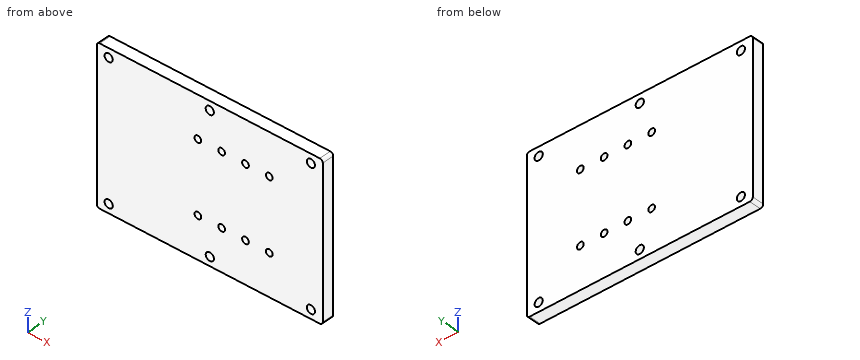
```python
from build123d import *

# Parameters (mm, degrees)
SKETCH1_W               = 482.6
SKETCH1_H               = 330.2
BOSS_EXTRUDE1_DEPTH     = 25.4
CUT_EXTRUDE1_DEPTH      = 294.477188211
CUT_EXTRUDE1_DEPTH_BACK = 294.477188211
SKETCH2_R               = 8.7376
CUT_EXTRUDE2_DEPTH      = 294.477188211
CUT_EXTRUDE2_DEPTH_BACK = 294.477188211
SKETCH4_R               = 7.1628
FILLET1_R               = 6.35


with BuildPart() as part:
    # Sketch1 → Boss-Extrude1 (new body)
    with BuildSketch(Plane(origin=(0, 0, 0), x_dir=(1, 0, 0), z_dir=(0, 1, 0))):
        Rectangle(SKETCH1_W, SKETCH1_H)
    extrude(amount=BOSS_EXTRUDE1_DEPTH)

    # Sketch2 → Cut-Extrude1 (cut, two sides: drawn at the far end of the back side and taken through both)
    with BuildSketch(Plane(origin=(0, 25.4, 0), x_dir=(1, 0, 0), z_dir=(0, 1, 0)).offset(-CUT_EXTRUDE1_DEPTH_BACK)):
        with Locations(Location((215.9, 146.05, 0), (0, 0, 270))):
            Circle(SKETCH2_R)
        with Locations(Location((-215.9, 146.05, 0), (0, 0, 270))):
            Circle(SKETCH2_R)
        with Locations(Location((215.9, -146.05, 0), (0, 0, 270))):
            Circle(SKETCH2_R)
        with Locations(Location((-215.9, -146.05, 0), (0, 0, 270))):
            Circle(SKETCH2_R)
        with Locations(Location((0, 146.05, 0), (0, 0, 270))):
            Circle(SKETCH2_R)
        with Locations(Location((0, -146.05, 0), (0, 0, 270))):
            Circle(SKETCH2_R)
    extrude(amount=CUT_EXTRUDE1_DEPTH + CUT_EXTRUDE1_DEPTH_BACK, mode=Mode.SUBTRACT)

    # Sketch4 → Cut-Extrude2 (cut, two sides: drawn at the far end of the back side and taken through both)
    with BuildSketch(Plane(origin=(0, 25.4, 0), x_dir=(1, 0, 0), z_dir=(0, 1, 0)).offset(-CUT_EXTRUDE2_DEPTH_BACK)):
        with Locations(Location((-25.4, 76.2, 0), (0, 0, 270))):
            Circle(SKETCH4_R)
        with Locations(Location((25.4, 76.2, 0), (0, 0, 270))):
            Circle(SKETCH4_R)
        with Locations(Location((76.2, 76.2, 0), (0, 0, 270))):
            Circle(SKETCH4_R)
        with Locations(Location((127, 76.2, 0), (0, 0, 270))):
            Circle(SKETCH4_R)
        with Locations(Location((127, -76.2, 0), (0, 0, 270))):
            Circle(SKETCH4_R)
        with Locations(Location((76.2, -76.2, 0), (0, 0, 270))):
            Circle(SKETCH4_R)
        with Locations(Location((25.4, -76.2, 0), (0, 0, 270))):
            Circle(SKETCH4_R)
        with Locations(Location((-25.4, -76.2, 0), (0, 0, 270))):
            Circle(SKETCH4_R)
    extrude(amount=CUT_EXTRUDE2_DEPTH + CUT_EXTRUDE2_DEPTH_BACK, mode=Mode.SUBTRACT)

    # Fillet1
    fillet1_edges = [part.edges().sort_by_distance(p)[0] for p in [
        (241.3, 12.7, 165.1),
        (-241.3, 12.7, 165.1),
        (-241.3, 12.7, -165.1),
        (241.3, 12.7, -165.1),
    ]]
    fillet(fillet1_edges, radius=FILLET1_R)


solid = part.part
```
CAD build for the part. Positions are in the model's coordinates, mm. Coordinates: 2 decimals unless noted, no trailing zeros. Order: outer loops, then holes, each group sorted by start corner. A loop starts at its lowest first (then second) coordinate and runs counter-clockwise, first axis right, second up. Notation, with made-up numbers: (-22, 36) -> (-10, 36) arc R27 cw to (-10, 68) -> close; hole circle Ø8 at (-5, -23.75). An arc over 180 degrees is marked (long way). Use one line per item in the form item = value. Start each with the question number.
1) Drop a flat-ended pin along its axis: pin 1 (13 mm diameter, centred on x = 76.2, z = 76.2, fed in from +Y). Give the stop position or say it passes through.
2) Band-saw the part on D-D on y = 7. State how many separate pieces and enclosed holes the cut face has, then the cut area to 3 significant figures.
3) Band-saw the part on C-C on z = -146.05. Give the cut face in (x, y), then the cut area to 3 significant figures.
4) Drill centre lines: L1, parallel to X at y = 4.25, z = 146.5; L2, parallel to Z at x = -25.4, y = 11; L3, parallel to X at y = 11, z = 76.2. Where is each one in solid material? Low to high. Write a range as [from, to].
5) Band-saw the part on B-B on x = 215.9. Give the cut face in (y, z).
6) Band-saw the part on A-A on z = -76.2. Give the cut face in (x, y), then the cut area to 3 significant figures.
Entries:
q1.pin_1 = through
q2.separate_pieces = 1
q2.enclosed_holes = 14
q2.area = 157,000 mm2
q3.outline = (-241.3, 0) -> (-224.64, 0) -> (-224.64, 25.4) -> (-241.3, 25.4) -> close; (-207.16, 0) -> (-8.74, 0) -> (-8.74, 25.4) -> (-207.16, 25.4) -> close; (8.74, 0) -> (207.16, 0) -> (207.16, 25.4) -> (8.74, 25.4) -> close; (224.64, 0) -> (241.3, 0) -> (241.3, 25.4) -> (224.64, 25.4) -> close
q3.area = 10,900 mm2
q4.L1 = [-241.3, -224.63], [-207.17, -8.73], [8.73, 207.17], [224.63, 241.3]
q4.L2 = [-165.1, -83.36], [-69.04, 69.04], [83.36, 165.1]
q4.L3 = [-241.3, -32.56], [-18.24, 18.24], [32.56, 69.04], [83.36, 119.84], [134.16, 241.3]
q5.outline = (0, -165.1) -> (25.4, -165.1) -> (25.4, -154.79) -> (0, -154.79) -> close; (0, -137.31) -> (25.4, -137.31) -> (25.4, 137.31) -> (0, 137.31) -> close; (0, 154.79) -> (25.4, 154.79) -> (25.4, 165.1) -> (0, 165.1) -> close
q6.outline = (-241.3, 0) -> (-32.56, 0) -> (-32.56, 25.4) -> (-241.3, 25.4) -> close; (-18.24, 0) -> (18.24, 0) -> (18.24, 25.4) -> (-18.24, 25.4) -> close; (32.56, 0) -> (69.04, 0) -> (69.04, 25.4) -> (32.56, 25.4) -> close; (83.36, 0) -> (119.84, 0) -> (119.84, 25.4) -> (83.36, 25.4) -> close; (134.16, 0) -> (241.3, 0) -> (241.3, 25.4) -> (134.16, 25.4) -> close
q6.area = 10,800 mm2
